For this review, take the finished solid that the model builds, in its own axes (mm). A direction names the side the tool comes from. Round coordinates to 2 decimals unless told otherwise and drop trailing zeros. Loops run counter-clockwise (first coordinate to the right, second up) from the corner with the lowest first, then second, coordinate; pieces in that order, holes last.
1. Consider section D-D on y = 10.75. State the section outline as (x, z) points.
2. Draft analysis for pull direction Y (two halves, no side actions). For faces 5 (the flat face through (19.75, 7, -10)), 6 (the flat face through (0, 9.75, -4)), 7 (the flat face through (18, 4.25, -9)), state which applies: released by +Y, released by -Y, zero draft, split by the parting line, or undercut.
3. To check wall thickness, follow line 1 along Z through (x, y) = (18.5, 5); line 2 along Y through (x, z) = (17.8, -15); line 3 along Z through (x, y) = (10.25, 9.75). State the ranges of each line that lie inside material, in increasing order.
4. Clearance check with flat-ended pins moving along their axes: pin 1 Ø6 at (y, z) = (4, -7.5) entering from +X; pin 2 Ø2 at (y, z) = (7.5, -2) entering from +X; pin 3 Ø1.2 at (x, z) = (0.5, -4.5) entering from -Y. State where each tip first meets the part, or that it passes through.
5. Consider section B-B on y = 7.25. State how many separate pieces and enclosed holes the cut face has, then the cut area to 3 significant figures.
6. Tool access review of faces 1 (the flat face through (0, 7.1, 0.5)), 2 (the flat face through (3.15, 7, -9)), 3 (the flat face through (20.14, 6.71, -1.97)), 4 (the flat face through (20.4, 3.75, -4.6)): name each direction out of +Z, -Z, +X, -X, +Y, -Y from which nothing blocks a thin tool from reaching the whole face with its end or side.
7. Consider section A-A on z = -15. State the section outline as (x, y) points, then the cut area to 3 significant figures.
from build123d import *

# Parameters (mm, degrees)
SKETCH_1_W          = 20.5
SKETCH_1_H          = 14.5
EXTRUDE_1_DEPTH     = 2
FILLET_1_R          = 1
SKETCH_2_W          = 18
SKETCH_2_H          = 11
EXTRUDE_2_DEPTH     = 11
SKETCH_3_W          = 2.5
SKETCH_3_H          = 11
EXTRUDE_3_DEPTH     = 0.5
SKETCH_4_W          = 2.5
SKETCH_4_H          = 11
EXTRUDE_4_DEPTH     = 0.5
SKETCH_5_R          = 0.3
CUT_EXTRUDE_1_DEPTH = 27.529464751
SKETCH_6_W          = 0.6
SKETCH_6_H          = 4
EXTRUDE_5_DEPTH     = 0.5
SKETCH_7_W          = 0.818024616
SKETCH_7_H          = 6
SKETCH_7_W_2        = 0.8
CUT_EXTRUDE_2_DEPTH = 4
SKETCH_8_W          = 0.6
SKETCH_8_H          = 5.5
EXTRUDE_6_DEPTH     = 11
CHAMFER_1_SIZE      = 1.2
SKETCH_9_R          = 1
CUT_EXTRUDE_3_DEPTH = 30.326651701
EXTRUDE_7_DEPTH     = 6
EXTRUDE_8_DEPTH     = 11
SKETCH_12_W         = 17.2
SKETCH_12_H         = 11.2
SKETCH_12_W_2       = 17
SKETCH_12_H_2       = 11
CUT_EXTRUDE_4_DEPTH = 10
SKETCH_13_W         = 17
SKETCH_13_H         = 0.1
CUT_EXTRUDE_5_DEPTH = 1


with BuildPart() as part:
    # 草图1 → 凸台-拉伸1 (new body)
    with BuildSketch(Plane.XY):
        with Locations((10.25, 7.25)):
            Rectangle(SKETCH_1_W, SKETCH_1_H)
    extrude(amount=EXTRUDE_1_DEPTH)

    # 圆角1
    fillet_1_edges = [part.edges().sort_by_distance(p)[0] for p in [
        (20.5, 7.25, 2),
        (10.25, 14.5, 2),
        (0, 7.25, 2),
        (10.25, 0, 2),
    ]]
    fillet(fillet_1_edges, radius=FILLET_1_R)

    # 草图2 → 凸台-拉伸2 (add)
    with BuildSketch(Plane(origin=(0, 0, 0), x_dir=(-1, 0, 0), z_dir=(0, 0, -1))):
        with Locations((-10.25, 7.25)):
            Rectangle(SKETCH_2_W, SKETCH_2_H)
    extrude(amount=EXTRUDE_2_DEPTH)

    # 草图3 → 凸台-拉伸3 (add)
    with BuildSketch(Plane(origin=(19.25, 0, 0), x_dir=(0, 0, -1), z_dir=(1, 0, 0))):
        with Locations((9.75, 7.25)):
            Rectangle(SKETCH_3_W, SKETCH_3_H)
    extrude(amount=EXTRUDE_3_DEPTH)

    # 草图4 → 凸台-拉伸4 (add)
    with BuildSketch(Plane.ZY.offset(-1.25)):
        with Locations((-9.75, 7.25)):
            Rectangle(SKETCH_4_W, SKETCH_4_H)
    extrude(amount=EXTRUDE_4_DEPTH)

    # 草图5 → 切除-拉伸1 (cut, through all)
    with BuildSketch(Plane(origin=(0, 12.75, 0), x_dir=(1, 0, 0), z_dir=(0, 1, 0))):
        with Locations(Location((10.25, 0.5, 0), (0, 0, 180))):
            Circle(SKETCH_5_R)
    extrude(amount=-CUT_EXTRUDE_1_DEPTH, mode=Mode.SUBTRACT)

    # 草图6 → 凸台-拉伸5 (add)
    with BuildSketch(Plane(origin=(0, 0, -11), x_dir=(-1, 0, 0), z_dir=(0, 0, -1))):
        with Locations((-18.45, 7.25)):
            Rectangle(SKETCH_6_W, SKETCH_6_H)
        with Locations((-17.05, 7.25)):
            Rectangle(SKETCH_6_W, SKETCH_6_H)
        with Locations((-10.95, 7.25)):
            Rectangle(SKETCH_6_W, SKETCH_6_H)
        with Locations((-9.55, 7.25)):
            Rectangle(SKETCH_6_W, SKETCH_6_H)
        with Locations((-3.45, 7.25)):
            Rectangle(SKETCH_6_W, SKETCH_6_H)
        with Locations((-2.05, 7.25)):
            Rectangle(SKETCH_6_W, SKETCH_6_H)
    extrude(amount=EXTRUDE_5_DEPTH)

    # 草图7 → 切除-拉伸2 (cut)
    with BuildSketch(Plane(origin=(0, 0, -11), x_dir=(-1, 0, 0), z_dir=(0, 0, -1))):
        with Locations((-17.740987692, 7.25)):
            Rectangle(SKETCH_7_W, SKETCH_7_H)
        with Locations((-10.25, 7.25)):
            Rectangle(SKETCH_7_W_2, SKETCH_7_H)
        with Locations((-2.75, 7.25)):
            Rectangle(SKETCH_7_W_2, SKETCH_7_H)
    extrude(amount=-CUT_EXTRUDE_2_DEPTH, mode=Mode.SUBTRACT)

    # 草图8 → 凸台-拉伸6 (add)
    with BuildSketch(Plane(origin=(0, 0, -7), x_dir=(-1, 0, 0), z_dir=(0, 0, -1))):
        with Locations((-17.75, 7.25)):
            Rectangle(SKETCH_8_W, SKETCH_8_H)
        with Locations((-10.25, 7.25)):
            Rectangle(SKETCH_8_W, SKETCH_8_H)
    extrude(amount=EXTRUDE_6_DEPTH)

    # 倒角1
    chamfer_1_edges = [part.edges().sort_by_distance(p)[0] for p in [
        (17.75, 4.5, -18),
        (17.75, 10, -18),
        (10.25, 4.5, -18),
        (10.25, 10, -18),
    ]]
    chamfer(chamfer_1_edges, length=CHAMFER_1_SIZE)

    # 草图9 → 切除-拉伸3 (cut, through all)
    with BuildSketch(Plane(origin=(18.05, 0, 0), x_dir=(0, 0, -1), z_dir=(1, 0, 0))):
        with Locations((15, 7.25)):
            Circle(SKETCH_9_R)
    extrude(amount=-CUT_EXTRUDE_3_DEPTH, mode=Mode.SUBTRACT)

    # 草图10 → 凸台-拉伸7 (add)
    with BuildSketch(Plane(origin=(0, 3.75, 0), x_dir=(-1, 0, 0), z_dir=(0, -1, 0))):
        Polygon((-19.25, 0), (-19.55, 0), (-20.75, 4), (-19.75, 8.5), (-19.25, 8.5), (-20.25, 4), align=None)
        Polygon((-1.25, 0), (-0.95, 0), (0.25, 4), (-0.75, 8.5), (-1.25, 8.5), (-0.25, 4), align=None)
    extrude(amount=-EXTRUDE_7_DEPTH)

    # 草图11 → 凸台-拉伸8 (add)
    with BuildSketch(Plane.XZ.offset(-1.75)):
        with BuildLine():
            Line((18.75, 2), (1.75, 2))
            ThreePointArc((1.75, 2), (2.005105989, 4.934028723), (2.762767594, 7.78))
            ThreePointArc((2.762767594, 7.78), (10.25, 3.489364109), (18.75, 2))
        make_face()
    extrude(amount=-EXTRUDE_8_DEPTH)

    # 草图12 → 切除-拉伸4 (cut)
    with BuildSketch(Plane.XY.offset(2)):
        with Locations((10.25, 7.25)):
            Rectangle(SKETCH_12_W, SKETCH_12_H)
        with Locations((10.25, 7.25)):
            Rectangle(SKETCH_12_W_2, SKETCH_12_H_2, mode=Mode.SUBTRACT)
    extrude(amount=-CUT_EXTRUDE_4_DEPTH, mode=Mode.SUBTRACT)

    # 草图13 → 切除-拉伸5 (cut)
    with BuildSketch(Plane.XY.offset(2)):
        with Locations((10.25, 1.8)):
            Rectangle(SKETCH_13_W, SKETCH_13_H)
        with Locations((10.25, 12.7)):
            Rectangle(SKETCH_13_W, SKETCH_13_H)
    extrude(amount=-CUT_EXTRUDE_5_DEPTH, mode=Mode.SUBTRACT)


solid = part.part
Resolved:
1. outline: (0, 0) - (1.25, 0) - (1.25, -8.5) - (0.75, -8.5) - (0.75, -11) - (19.75, -11) - (19.75, -8.5) - (19.25, -8.5) - (19.25, 0) - (20.5, 0) - (20.5, 1) arc R1 ccw to (19.5, 2) - (18.85, 2) - (18.85, -8) - (18.75, -8) - (18.75, 2) arc R25 cw to (2.76, 7.78) arc R17 ccw to (1.75, 2) - (1.75, -8) - (1.65, -8) - (1.65, 2) - (1, 2) arc R1 ccw to (0, 1) - close; hole circle Ø0.6 at (10.25, -0.5)
2. face 5: zero draft
2. face 6: released by +Y
2. face 7: undercut
3. line 1: z = -11 to 2
3. line 2: y = 4.5 to 6.25, 8.25 to 10
3. line 3: z = -17.05 to -0.8, -0.2 to 3.49
4. pin 1: stops at x = 20.64
4. pin 2: stops at x = 20.45
4. pin 3: stops at y = 3.75
5. separate pieces: 3
5. enclosed holes: 3
5. area: 283 mm2
6. face 1: +Z, -X, +Y, -Y
6. face 2: -Z
6. face 3: +X, +Y, -Y
6. face 4: +X, -Y
7. outline: (9.95, 4.5) - (10.55, 4.5) - (10.55, 6.25) - (9.95, 6.25) - close; (9.95, 8.25) - (10.55, 8.25) - (10.55, 10) - (9.95, 10) - close; (17.45, 4.5) - (18.05, 4.5) - (18.05, 6.25) - (17.45, 6.25) - close; (17.45, 8.25) - (18.05, 8.25) - (18.05, 10) - (17.45, 10) - close
7. area: 4.20 mm2
